Source: CAD feature listing. Evaluate the final solid. Frame: model axes, mm. Round coordinates to 2 decimals unless told otherwise and drop trailing zeros. Write each loop counter-clockwise with the first axis right and the second up, starting at its lowest first coordinate (ties: lowest second). Pieces come first, ordered by that corner, then holes. Notation, with made-up numbers: M 69.5,44.25 L 112.5,44.25 A8 cw 112.5,57.25 Z; hole C 44.25,-25.5 d6. An arc over 180 degrees is marked long. Put each result on its own line as item: value. Start each with the question number.
```python
from build123d import *

# Parameters (mm, degrees)
F1_DEPTH = 6.35
F3_DEPTH = 25.4


with BuildPart() as f1:
    # F0 (on Front) → F1 (new body)
    with BuildSketch(Plane.XZ):
        with BuildLine():
            ThreePointArc((119.0625, 77.7875), (115.342756, 86.767756), (106.3625, 90.4875))
            Line((106.3625, 90.4875), (-106.3625, 90.4875))
            ThreePointArc((-106.3625, 90.4875), (-115.342756, 86.767756), (-119.0625, 77.7875))
            Line((-119.0625, 77.7875), (-119.0625, -77.7875))
            ThreePointArc((-119.0625, -77.7875), (-115.342756, -86.767756), (-106.3625, -90.4875))
            Line((-106.3625, -90.4875), (106.3625, -90.4875))
            ThreePointArc((106.3625, -90.4875), (115.342756, -86.767756), (119.0625, -77.7875))
            Line((119.0625, -77.7875), (119.0625, 77.7875))
        make_face()
        with BuildLine():
            Line((119.0625, 90.4875), (106.3625, 90.4875))
            ThreePointArc((106.3625, 90.4875), (115.342756, 86.767756), (119.0625, 77.7875))
            Line((119.0625, 77.7875), (119.0625, 90.4875))
        make_face()
        with BuildLine():
            ThreePointArc((-119.0625, 77.7875), (-115.342756, 86.767756), (-106.3625, 90.4875))
            Line((-106.3625, 90.4875), (-119.0625, 90.4875))
            Line((-119.0625, 90.4875), (-119.0625, 77.7875))
        make_face()
        with BuildLine():
            Line((119.0625, -90.4875), (119.0625, -77.7875))
            ThreePointArc((119.0625, -77.7875), (115.342756, -86.767756), (106.3625, -90.4875))
            Line((106.3625, -90.4875), (119.0625, -90.4875))
        make_face()
        with BuildLine():
            ThreePointArc((-106.3625, -90.4875), (-115.342756, -86.767756), (-119.0625, -77.7875))
            Line((-119.0625, -77.7875), (-119.0625, -90.4875))
            Line((-119.0625, -90.4875), (-106.3625, -90.4875))
        make_face()
    extrude(amount=F1_DEPTH)

    # F2 (on face) → F3 (cut)
    with BuildSketch(Plane(origin=(0, 0, 0), x_dir=(-1, 0, 0), z_dir=(0, 1, 0))):
        Polygon((-14.2875, -90.4875), (119.0625, -90.4875), (119.0625, -46.0375), align=None)
    extrude(amount=-F3_DEPTH, mode=Mode.SUBTRACT)


solid = f1.part
```
(1) Section query C-C (x = -14.5). Return loops of the section in (y, z).
(2) Contact query for a flat-ended pin moving along its axis: P1, Ø5, axis at x = 40, z = -21.5, coming from the +Y side. Output: stop coordinate, or through.
(3) Section query A-A (y = -2). Return loops of the section in (x, z), and give its area (3 significant figures).
(4) Ray query, line 1 along Z through (x, y) = (-21, -3.5) (1 decimal); line 2 along Z through (x, y) = (-101, -4). Return the intervals inside material, ascending.
Entries:
1. outline: M -6.35,-80.89 L 0,-80.89 L 0,90.49 L -6.35,90.49 Z
2. P1: y = 0
3. outline: M -119.06,-46.04 L 14.29,-90.49 L 119.06,-90.49 L 119.06,90.49 L -119.06,90.49 Z
3. area: 40,100 mm2
4. line 1: -78.7 to 90.5
4. line 2: -52.06 to 90.49
